Here's how the part is built. I have some questions about the finished solid (model axes, mm). Face numbers are marked on the shaded views. A direction names the side the tool comes from. Give positions to 0.01 mm unless a question says otherwise; leave off trailing zeros. Write each loop counter-clockwise with the first axis right and the second up, starting at its lowest first coordinate (ties: lowest second). Pieces come first, ordered by that corner, then holes. Notation, with made-up numbers: (87, 34) -> (140, 34) arc R34 cw to (140, 67) -> close; hole circle Ø4 at (32, 51). An arc over 180 degrees is marked (long way). Use one line per item in the form item = value.
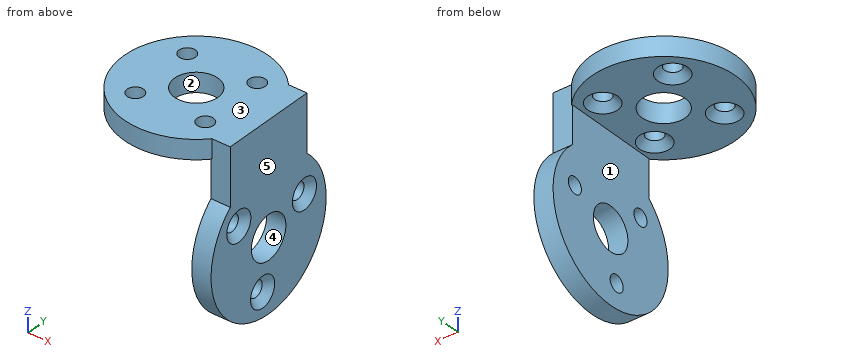
```python
from build123d import *

# Parameters (mm, degrees)
ESQUISSE1_R                                    = 4.5
ESQUISSE1_R_2                                  = 1.5
BOSS_EXTRU_1_DEPTH                             = 4
ESQUISSE3_R                                    = 4.5
ESQUISSE3_R_2                                  = 1.500083245
BOSS_EXTRU_2_DEPTH                             = 4
FRAISAGE_POUR_VIS_T_TE_FRAIS_E_M31_D           = 3.4
FRAISAGE_POUR_VIS_T_TE_FRAIS_E_M31_CSINK_D     = 6.3
FRAISAGE_POUR_VIS_T_TE_FRAIS_E_M31_CSINK_ANGLE = 90
FRAISAGE_POUR_VIS_T_TE_FRAIS_E_M32_D           = 3.4
FRAISAGE_POUR_VIS_T_TE_FRAIS_E_M32_CSINK_D     = 6.3
FRAISAGE_POUR_VIS_T_TE_FRAIS_E_M32_CSINK_ANGLE = 90


with BuildPart() as part:
    # Esquisse1 → Boss.-Extru.1 (new body)
    with BuildSketch(Plane.XY):
        with BuildLine():
            Line((11.180339887, 10), (15, 10))
            Line((15, 10), (15, -10))
            Line((15, -10), (11.180339887, -10))
            ThreePointArc((11.180339887, -10), (-15, 0), (11.180339887, 10))
        make_face()
        Circle(ESQUISSE1_R, mode=Mode.SUBTRACT)
        with Locations((-7.303420571, 6.830816054)):
            Circle(ESQUISSE1_R_2, mode=Mode.SUBTRACT)
        with Locations((6.830816054, 7.303420571)):
            Circle(ESQUISSE1_R_2, mode=Mode.SUBTRACT)
        with Locations((7.303420571, -6.830816054)):
            Circle(ESQUISSE1_R_2, mode=Mode.SUBTRACT)
        with Locations((-6.830816054, -7.303420571)):
            Circle(ESQUISSE1_R_2, mode=Mode.SUBTRACT)
    extrude(amount=BOSS_EXTRU_1_DEPTH)

    # Esquisse3 → Boss.-Extru.2 (add)
    with BuildSketch(Plane(origin=(15, 0, 0), x_dir=(0, 0, -1), z_dir=(1, 0, 0))):
        with BuildLine():
            Line((0, 10), (7.819660113, 10))
            ThreePointArc((7.819660113, 10), (34, 0), (7.819660113, -10))
            Line((7.819660113, -10), (0, -10))
            Line((0, -10), (0, 10))
        make_face()
        with Locations((19, 0)):
            Circle(ESQUISSE3_R, mode=Mode.SUBTRACT)
        with Locations((15.416309522, 9.335800049)):
            Circle(ESQUISSE3_R_2, mode=Mode.SUBTRACT)
        with Locations((28.876885246, -1.564333031)):
            Circle(ESQUISSE3_R_2, mode=Mode.SUBTRACT)
        with Locations((12.706805232, -7.771467018)):
            Circle(ESQUISSE3_R_2, mode=Mode.SUBTRACT)
    extrude(amount=-BOSS_EXTRU_2_DEPTH)

    # Fraisage pour vis à tête fraisée M31 (through all)
    with Locations(Plane(origin=(0, 0, 0), x_dir=(-1, 0, 0), z_dir=(0, 0, -1))):
        with Locations((-6.830816054, 7.303420571), (7.303420571, 6.830816054), (6.830816054, -7.303420571), (-7.303420571, -6.830816054)):
            CounterSinkHole(FRAISAGE_POUR_VIS_T_TE_FRAIS_E_M31_D / 2, FRAISAGE_POUR_VIS_T_TE_FRAIS_E_M31_CSINK_D / 2, counter_sink_angle=FRAISAGE_POUR_VIS_T_TE_FRAIS_E_M31_CSINK_ANGLE)

    # Fraisage pour vis à tête fraisée M32 (through all)
    with Locations(Plane(origin=(15, 0, 0), x_dir=(0, 0, -1), z_dir=(1, 0, 0))):
        with Locations((15.416309522, 9.335800049), (28.876885246, -1.564333031), (12.706805232, -7.771467018)):
            CounterSinkHole(FRAISAGE_POUR_VIS_T_TE_FRAIS_E_M32_D / 2, FRAISAGE_POUR_VIS_T_TE_FRAIS_E_M32_CSINK_D / 2, counter_sink_angle=FRAISAGE_POUR_VIS_T_TE_FRAIS_E_M32_CSINK_ANGLE)


solid = part.part
```
Q1. I want a section at C-C, the plane y = 2.75. Write out the boundary of the cut face in (x, z).
Result set:
outline = (-14.75, 0) -> (-3.56, 0) -> (-3.56, 4) -> (-14.75, 4) -> close; (3.56, 0) -> (11, 0) -> (11, -15.44) -> (15, -15.44) -> (15, 4) -> (3.56, 4) -> close; (11, -33.75) -> (15, -33.75) -> (15, -22.56) -> (11, -22.56) -> close
Q2. Will these pins go through, and if not, where does the flat tip stop? pin 1 Ø4.5 at (y, z) = (-7.77, -12.71) entering from -X; pin 2 Ø3 at (x, y) = (6.83, 7.3) entering from +Z; pin 3 Ø5.5 at (y, z) = (9.34, -15.42) entering from +X; pin 4 Ø2 at (x, z) = (13.5, 0) entering from +Y.
Result set:
pin_1 = 11
pin_2 = through
pin_3 = 14.61
pin_4 = 10
Q3. I want a section at B-B, the plane z = -23. Write out the boundary of the cut face in (x, y), and give its area (3 significant figures).
Result set:
outline = (11, -14.46) -> (15, -14.46) -> (15, -2.06) -> (11, -2.06) -> close; (11, 2.06) -> (15, 2.06) -> (15, 14.46) -> (11, 14.46) -> close
area = 99.2 mm2
Q4. If I drill on line 1 along Z through (x, y) = (-4, -5); line 2 along X through (y, z) = (7.5, -12.5); line 3 along Z through (x, y) = (11.5, -13.25), over which ranges is the centre line in solid material (lowest first)? Write a range as from..to.
Result set:
line_1 = 0..4
line_2 = 11..15
line_3 = -26.03..-11.97
Q5. If we mould it in two halves opening along Z, with no side actions, what happens to the marked faces 3, 4 and 5? For each: +Z half, -Z half, draft (parallel to the pull), parting line (faces both ways), or undercut.
Result set:
face_3 = +Z half
face_4 = undercut
face_5 = draft
Q6. I want a section at D-D, the plane x = 12.25. Write out the boundary of the cut face in (y, z), and give its area (3 significant figures).
Result set:
outline = (-10, -7.82) arc R15 ccw (long way) to (10, -7.82) -> (10, 4) -> (-10, 4) -> close; hole circle Ø3.4 at (-7.77, -12.71); hole circle Ø9 at (0, -19); hole circle Ø3.4 at (-1.56, -28.88); hole circle Ø3.4 at (9.34, -15.42)
area = 800 mm2
Q7. I want a section at A-A, the plane x = 0. Write out the boundary of the cut face in (y, z), and give its area (3 significant figures).
Result set:
outline = (-15, 0) -> (-4.5, 0) -> (-4.5, 4) -> (-15, 4) -> close; (4.5, 0) -> (15, 0) -> (15, 4) -> (4.5, 4) -> close
area = 84.0 mm2
Q8. Which directions (+Z, -Z, +X, -X, +Y, -Y) give clear straight access to the entire face, cutting with the end or side of a thin tool? Please do the marked faces 1 and 2.
Result set:
face_1 = -Z, -X, +Y, -Y
face_2 = +Z, -Z
